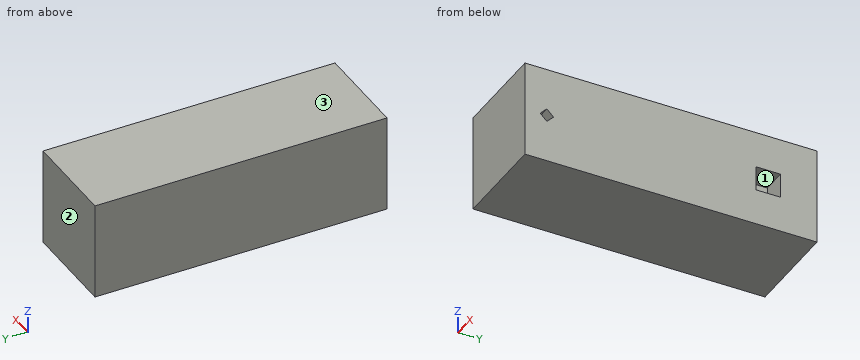
from build123d import *

# Parameters (mm, degrees)
F0_W     = 32
F0_H     = 96
F1_DEPTH = 32
F2_W     = 8.1
F2_H     = 8.1
F3_DEPTH = 8.1
F5_DEPTH = 4.1


with BuildPart() as f1:
    # F0 (on Top) → F1 (new body)
    with BuildSketch(Plane.XY):
        Rectangle(F0_W, F0_H)
    extrude(amount=F1_DEPTH)

    # F2 (on face) → F3 (cut)
    with BuildSketch(Plane.YZ.offset(16)):
        with Locations((31.95, 15.95)):
            Rectangle(F2_W, F2_H)
    extrude(amount=-F3_DEPTH, mode=Mode.SUBTRACT)

    # F4 (on face) → F5 (cut)
    with BuildSketch(Plane.YZ.offset(16)):
        Polygon((-38.615938, 16), (-40.807969, 18.192031), (-43, 16), (-40.807969, 13.807969), align=None)
    extrude(amount=-F5_DEPTH, mode=Mode.SUBTRACT)


solid = f1.part
Design review of the part built by this model. Coordinates are the model's own, in mm. Face numbers are marked on the shaded views. Coordinates: 2 decimals unless noted, no trailing zeros. Write each loop counter-clockwise with the first axis right and the second up, starting at its lowest first coordinate (ties: lowest second). Pieces come first, ordered by that corner, then holes. Notation, with made-up numbers: (-14, 24.25) - (42, 24.25) arc R14 ccw to (42, 33.25) - close; hole circle Ø7 at (29, 19). An arc over 180 degrees is marked (long way). One line per item, written item: value.
1) Insertion check: pin 1 (2.5 mm diameter, centred on y = 33, z = 16.5, fed in from +X). The pin has a flat end and moves straight along its axis. Give the tip position at first contact, or say it passes through.
Answer sheet:
pin 1: stops at x = 7.9
2) Add section B-B (z = 15). State the section outline as (x, y) points, plus the area to 3 significant figures.
Answer sheet:
outline: (-16, -48) - (16, -48) - (16, -42) - (11.9, -42) - (11.9, -39.62) - (16, -39.62) - (16, 27.9) - (7.9, 27.9) - (7.9, 36) - (16, 36) - (16, 48) - (-16, 48) - close
area: 3,000 mm2
3) To check wall thickness, follow probe 1 along Y at (x, z) = (12, 19); probe 2 along X at (y, z) = (30, 16.5). State the ranges of each line that lie inside material, in increasing order.
Answer sheet:
probe 1: y = -48 to 27.9, 36 to 48
probe 2: x = -16 to 7.9
4) Add section A-A (x = 11). State the section outline as (y, z) points, plus the area to 3 significant figures.
Answer sheet:
outline: (-48, 0) - (48, 0) - (48, 32) - (-48, 32) - close; hole (27.9, 11.9) - (36, 11.9) - (36, 20) - (27.9, 20) - close
area: 3,010 mm2
5) Mouldability with a two-part tool opening along Z and no side actions: class the marked faces 1, 2 and 3 as +Z half, -Z half, draft (parallel to the pull), parting line (faces both ways), or undercut.
Answer sheet:
face 1: undercut
face 2: draft
face 3: +Z half
